For this review, take the finished solid that the model builds, in its own axes (mm). A direction names the side the tool comes from. Round coordinates to 2 decimals unless told otherwise and drop trailing zeros. Order: outer loops, then holes, each group sorted by start corner. A loop starts at its lowest first (then second) coordinate and runs counter-clockwise, first axis right, second up. Notation, with made-up numbers: (-11.75, -26.5) - (34.25, -26.5) arc R37 ccw to (34.25, 10.5) - close; hole circle Ø8 at (27.25, 39). An arc over 180 degrees is marked (long way). Write each question's results on one line, items separated by ' | '. Start each with the question number.
(1) Take a section at A-A, the plane z = -16. Give the boundary of the cut face in (x, y), plus the area to 3 significant figures.
(2) Draft analysis for pull direction X (two halves, no side actions). For faces 4 (the flat face through (10, 82, 66)), 5 (the flat face through (-5, 38, 93)), 6 (the cylindrical face through (1.03, 74.68, -76.27)), state which applies: pulls with the +X half, pulls with the -X half, needs draft (parallel to the pull), parting line crosses it, or undercut.
(3) For L1, parallel to Y at x = -8, z = 0 (3 decimals); L2, parallel to Y at x = 2.5, z = 0 (3 decimals); L3, parallel to Y at x = -3.65, z = 0 (3 decimals), list the stretches that pass through material, from the lowest coordinate up. Write a range as from..to.
(4) Insertion check: pin 1 Ø1 at (x, z) = (2, -35) entering from +Y; pin 2 Ø8 at (x, y) = (3.5, -73) entering from +Z; pin 3 Ø2 at (x, z) = (-7.5, 64.5) entering from -Y; pin 4 Ø3 at (y, z) = (54.03, -93.58) entering from -X. Each pin has a flat end and moves straight along its axis. Give the tip position at first contact, or say it passes through.
(5) For faces 1 (the cylindrical face through (-7.54, -31.54, -100.15)), 2 (the cylindrical face through (0, -68, 74)), 3 (the flat face through (5, 93, -38)), list the 3-axis set-ups (+Z, -Z, +X, -X, +Y, -Y) from which the entire face can be reached by the end or side of a thin tool; tool diameter is ignored.
(6) Take a section at B-B, the plane y = 39.5. Give the boundary of the cut face in (x, z).
```python
from build123d import *

# Parameters (mm, degrees)
TAP_DRILL_FOR_4_40_TAP2_D     = 2.2606
TAP_DRILL_FOR_4_40_TAP2_DEPTH = 8.89
TAP_DRILL_FOR_4_40_TAP2_TIP   = 0.679152758
TAP_DRILL_FOR_4_40_TAP3_D     = 2.2606
TAP_DRILL_FOR_4_40_TAP3_DEPTH = 8.89
TAP_DRILL_FOR_4_40_TAP3_TIP   = 0.679152758
SKETCH9_R                     = 1.524
CUT_EXTRUDE1_DEPTH            = 8.89
CIRPATTERN1_COUNT             = 6
TAP_DRILL_FOR_4_40_TAP1_D     = 2.2606
TAP_DRILL_FOR_4_40_TAP1_DEPTH = 6.35
TAP_DRILL_FOR_4_40_TAP1_TIP   = 0.679152758


with BuildPart() as part:
    # Sketch3 → Revolve1 (revolve)
    with BuildSketch(Plane(origin=(0, 0, 0), x_dir=(1, 0, 0), z_dir=(0, 1, 0)), mode=Mode.PRIVATE) as revolve1_sk:
        Polygon((-10, -111.125), (10, -111.125), (10, -105), (5, -105), (5, -100), (1.5875, -100), (1.5875, -100.5), (-1.5875, -100.5), (-1.5875, -100), (-5, -100), (-5, -105), (-10, -105), align=None)
    revolve(revolve1_sk.sketch.rotate(Axis((0, 0, 0), (-1, 0, 0)), 180), axis=Axis((0, 0, 0), (-1, 0, 0)))

    # Tap Drill for _4-40 Tap2
    with Locations(Plane(origin=(5, -102.5, 0), x_dir=(0, 0, 1), z_dir=(1, 0, 0))):
        with Locations((0, 0), (-88.767603888, -51.25), (88.767603888, -51.25), (88.767603888, -153.75), (0, -205), (-88.767603888, -153.75)):
            Hole(TAP_DRILL_FOR_4_40_TAP2_D / 2, depth=TAP_DRILL_FOR_4_40_TAP2_DEPTH)
            with Locations((0, 0, -(TAP_DRILL_FOR_4_40_TAP2_DEPTH + TAP_DRILL_FOR_4_40_TAP2_TIP / 2))):  # 118° drill point
                Cone(0, TAP_DRILL_FOR_4_40_TAP2_D / 2, TAP_DRILL_FOR_4_40_TAP2_TIP, mode=Mode.SUBTRACT)

    # Tap Drill for _4-40 Tap3
    with Locations(Plane(origin=(-5, -88.767603888, 51.25), x_dir=(0, 0, -1), z_dir=(-1, 0, 0))):
        with Locations((0, 0), (-51.25, -88.767603888), (102.5, -177.535207776), (0, -177.535207776), (153.75, -88.767603888), (102.5, 0)):
            Hole(TAP_DRILL_FOR_4_40_TAP3_D / 2, depth=TAP_DRILL_FOR_4_40_TAP3_DEPTH)
            with Locations((0, 0, -(TAP_DRILL_FOR_4_40_TAP3_DEPTH + TAP_DRILL_FOR_4_40_TAP3_TIP / 2))):  # 118° drill point
                Cone(0, TAP_DRILL_FOR_4_40_TAP3_D / 2, TAP_DRILL_FOR_4_40_TAP3_TIP, mode=Mode.SUBTRACT)

    # Sketch9 → Cut-Extrude1 (cut)
    with BuildSketch(Plane(origin=(0, 107.338507446, 28.761266387), x_dir=(-1, 0, 0), z_dir=(0, 0.9659258262890681, 0.25881904510252135))):
        with Locations(Location((0, 0, 0), (0, 0, 90))):
            Circle(SKETCH9_R)
    cut_extrude1 = extrude(amount=-CUT_EXTRUDE1_DEPTH, mode=Mode.SUBTRACT)

    # CirPattern1: Cut-Extrude1 ×6 about axis
    cirpattern1_axis = Axis((0, 0, 0), (1, 0, 0))
    for i in range(1, CIRPATTERN1_COUNT):
        add(cut_extrude1.rotate(cirpattern1_axis, i * 360 / CIRPATTERN1_COUNT), mode=Mode.SUBTRACT)

    # Tap Drill for _4-40 Tap1
    with Locations(Plane(origin=(-10, 108.0625, 0), x_dir=(0, 0, -1), z_dir=(-1, 0, 0))):
        with Locations((0, 0), (-93.584870196, 54.03125), (-93.584870196, 162.09375), (0, 216.125), (93.584870196, 162.09375), (93.584870196, 54.03125)):
            Hole(TAP_DRILL_FOR_4_40_TAP1_D / 2, depth=TAP_DRILL_FOR_4_40_TAP1_DEPTH)
            with Locations((0, 0, -(TAP_DRILL_FOR_4_40_TAP1_DEPTH + TAP_DRILL_FOR_4_40_TAP1_TIP / 2))):  # 118° drill point
                Cone(0, TAP_DRILL_FOR_4_40_TAP1_D / 2, TAP_DRILL_FOR_4_40_TAP1_TIP, mode=Mode.SUBTRACT)


solid = part.part
```
Results below:
1) outline: (-10, -109.97) - (10, -109.97) - (10, -103.77) - (5, -103.77) - (5, -98.71) - (1.59, -98.71) - (1.59, -99.22) - (-1.59, -99.22) - (-1.59, -98.71) - (-5, -98.71) - (-5, -103.77) - (-10, -103.77) - close; (-10, 103.77) - (-5, 103.77) - (-5, 98.71) - (-1.59, 98.71) - (-1.59, 99.22) - (1.59, 99.22) - (1.59, 98.71) - (5, 98.71) - (5, 103.77) - (10, 103.77) - (10, 109.97) - (-10, 109.97) - close | area: 346 mm^2
2) face 4: pulls with the +X half | face 5: pulls with the -X half | face 6: undercut
3) L1: y = -111.125..-109.193, -106.932..-105, 105..106.932, 109.193..111.125 | L2: y = -111.125..-103.63, -101.37..-100, 100..101.37, 103.63..111.125 | L3: y = -111.125..-109.193, -106.932..-103.63, -101.37..-100, 100..101.37, 103.63..106.932, 109.193..111.125
4) pin 1: stops at y = 105.63 | pin 2: stops at z = 87.11 | pin 3: stops at y = -91.19 | pin 4: stops at x = -10
5) face 1: -X | face 2: none | face 3: +X
6) outline: (-10, -103.87) - (10, -103.87) - (10, -97.29) - (5, -97.29) - (5, -91.87) - (1.59, -91.87) - (1.59, -92.41) - (-1.59, -92.41) - (-1.59, -91.87) - (-5, -91.87) - (-5, -97.29) - (-10, -97.29) - close; (-10, 97.29) - (-5, 97.29) - (-5, 91.87) - (-1.59, 91.87) - (-1.59, 92.41) - (1.59, 92.41) - (1.59, 91.87) - (5, 91.87) - (5, 97.29) - (10, 97.29) - (10, 103.87) - (-10, 103.87) - close
